```python
from build123d import *

# Parameters (mm, degrees)
F1_DEPTH = 50.8
F2_DEPTH = 12.7
F4_DEPTH = 6.35


with BuildPart() as f1:
    # F0 (on Top) → F1 (new body)
    with BuildSketch(Plane.XY):
        with BuildLine():
            Line((33.810558, 27.093243), (38.079627, 27.093243))
            Line((38.079627, 27.093243), (38.079627, 17.69675))
            ThreePointArc((38.079627, 17.69675), (53.823516, 11.175418), (60.344848, -4.568471))
            ThreePointArc((60.344848, -4.568471), (53.823516, -20.312359), (38.079627, -26.833692))
            Line((38.079627, -26.833692), (38.079627, -36.230184))
            Line((38.079627, -36.230184), (33.810558, -36.230184))
            ThreePointArc((33.810558, -36.230184), (59.106989, -28.62131), (70.027851, -4.568471))
            ThreePointArc((70.027851, -4.568471), (59.106989, 19.484369), (33.810558, 27.093243))
        make_face()
        with BuildLine():
            Line((38.079627, 17.69675), (38.079627, 27.093243))
            Line((38.079627, 27.093243), (33.810558, 27.093243))
            ThreePointArc((33.810558, 27.093243), (6.131402, -4.568471), (33.810558, -36.230184))
            Line((33.810558, -36.230184), (38.079627, -36.230184))
            Line((38.079627, -36.230184), (38.079627, -26.833692))
            ThreePointArc((38.079627, -26.833692), (15.814406, -4.568471), (38.079627, 17.69675))
        make_face()
    extrude(amount=F1_DEPTH)

    # F0 (on Top) → F2 (join)
    with BuildSketch(Plane.XY):
        with BuildLine():
            Line((33.810558, 27.093243), (38.079627, 27.093243))
            Line((38.079627, 27.093243), (38.079627, 17.69675))
            ThreePointArc((38.079627, 17.69675), (53.823516, 11.175418), (60.344848, -4.568471))
            ThreePointArc((60.344848, -4.568471), (53.823516, -20.312359), (38.079627, -26.833692))
            Line((38.079627, -26.833692), (38.079627, -36.230184))
            Line((38.079627, -36.230184), (33.810558, -36.230184))
            ThreePointArc((33.810558, -36.230184), (59.106989, -28.62131), (70.027851, -4.568471))
            ThreePointArc((70.027851, -4.568471), (59.106989, 19.484369), (33.810558, 27.093243))
        make_face()
        with BuildLine():
            ThreePointArc((33.810558, -36.230184), (6.131402, -4.568471), (33.810558, 27.093243))
            Line((33.810558, 27.093243), (-38.079627, 27.093243))
            Line((-38.079627, 27.093243), (-38.079627, -36.230184))
            Line((-38.079627, -36.230184), (33.810558, -36.230184))
        make_face()
    extrude(amount=F2_DEPTH)

    # F3 (on Front) → F4 (join, symmetric)
    with BuildSketch(Plane.XZ):
        Polygon((6.229152, 13.422799), (4.844896, 36.124598), (-17.856903, 13.422799), align=None)
    extrude(amount=F4_DEPTH, both=True)


solid = f1.part
```
Here's how the part is built. I have some questions about the finished solid (model axes, mm). A direction names the side the tool comes from. Coordinates: 2 decimals unless noted, no trailing zeros. Write each loop counter-clockwise with the first axis right and the second up, starting at its lowest first coordinate (ties: lowest second). Pieces come first, ordered by that corner, then holes. Notation, with made-up numbers: (10, -25.5) -> (20, -25.5) arc R23 cw to (20, -13.5) -> close; hole circle Ø3 at (14, 30). An arc over 180 degrees is marked (long way). Use a Markdown table: item, result. Add a question column.
(1) We'd pull the mould along X, two halves only. Please class faces 5 (the flat face through (-1, -6.35, 22)), 6 (the flat face through (-38.08, -4, 6)), 7 (the flat face through (5.547, -0.089, 24.615)): +X half, -X half, draft (parallel to the pull), parting line (faces both ways), or undercut.
(2) If we section it at A-A, the plane z = 18: Write out the boundary of the cut face in (x, y).
(3) If we section it at C-C, the plane z = 7: Write out the boundary of the cut face in (x, y), and give its area (3 significant figures).
(4) If we section it at B-B, the plane y = 3.5: Write out the boundary of the cut face in (x, z).
(5) If we section it at D-D, the plane y = -21: Write out the boundary of the cut face in (x, z).
(6) Please list where these lines run through material, in increasing order: line 1 (X direction, y = 2, z = 15); line 2 (X direction, y = -5.5, z = 22.5); line 3 (X direction, y = 3, z = 7).
(7) I'm going to push flat-ended pins straight in: P1, Ø8, axis at x = 33.5, z = 15, coming from the -Y side; P2, Ø4, axis at y = 3, z = 22.5, coming from the -X side; P3, Ø25, axis at x = -3, z = 22.5, coming from the -Y side; P4, Ø4, axis at x = -5.5, y = 10.5, coming from the -Z side. Where does each tip first touch, or does it pass through?
(8) For faces 1 (the flat face through (-2, 27.093, 6)), 2 (the flat face through (-6, 0, 13.423)), 3 (the flat face through (-1, 6.35, 22)), 4 (the flat face through (-3, -36.23, 6)), which set-ups out of +Z, -Z, +X, -X, +Y, -Y let a thin tool reach every point of the face, with its end or its side?
Outcome:
| question | item | result |
|---|---|---|
| 1 | face 5 | draft |
| 1 | face 6 | -X half |
| 1 | face 7 | undercut |
| 2 | outline | (-13.28, -6.35) -> (5.95, -6.35) -> (5.95, 6.35) -> (-13.28, 6.35) -> close; circle Ø63.9 at (38.08, -4.57); hole (38.08, 17.7) arc R22.27 ccw (long way) to (60.34, -4.57) arc R22.27 ccw to start |
| 3 | outline | (-38.08, -36.23) -> (33.81, -36.23) arc R31.95 ccw (long way) to (33.81, 27.09) -> (-38.08, 27.09) -> close; hole (38.08, 17.7) arc R22.27 ccw (long way) to (60.34, -4.57) arc R22.27 ccw to start |
| 3 | area | 4,870 mm^2 |
| 4 | outline | (-38.08, 0) -> (17.33, 0) -> (17.33, 50.8) -> (7.17, 50.8) -> (7.17, 12.7) -> (-38.08, 12.7) -> close; (-17.86, 13.42) -> (6.23, 13.42) -> (4.84, 36.12) -> close; (58.83, 0) -> (68.99, 0) -> (68.99, 50.8) -> (58.83, 50.8) -> close |
| 5 | outline | (-38.08, 0) -> (23.05, 0) -> (23.05, 50.8) -> (10.68, 50.8) -> (10.68, 12.7) -> (-38.08, 12.7) -> close; (53.1, 0) -> (65.48, 0) -> (65.48, 50.8) -> (53.1, 50.8) -> close |
| 6 | line 1 | x = -16.28 to 6.13, 6.81 to 16.81, 59.35 to 69.35 |
| 6 | line 2 | x = -8.78 to 5.68, 6.14 to 15.83, 60.33 to 70.01 |
| 6 | line 3 | x = -38.08 to 17.14, 59.02 to 69.12 |
| 7 | P1 | stops at y = -36.51 |
| 7 | P2 | stops at x = -10.78 |
| 7 | P3 | stops at y = -36.23 |
| 7 | P4 | stops at z = 0 |
| 8 | face 1 | +Z, -Z, -X, +Y |
| 8 | face 2 | -X, +Y, -Y |
| 8 | face 3 | +Z, -X, +Y |
| 8 | face 4 | +Z, -Z, -X, -Y |
